Source: CAD feature listing. Evaluate the final solid. Frame: model axes, mm. A direction names the side the tool comes from. Coordinates: 2 decimals unless noted, no trailing zeros. Order: outer loops, then holes, each group sorted by start corner. A loop starts at its lowest first (then second) coordinate and runs counter-clockwise, first axis right, second up.
Item 1: Contact query for flat-ended pins moving along their axis: P1, Ø5.5, axis at x = 21, y = -2, coming from the +Z side; P2, Ø5, axis at x = -20.5, z = -1.5, coming from the -Y side; P3, Ø5, axis at y = -6.5, z = 3, coming from the +X side; P4, Ø5, axis at x = 11.5, y = -8, coming from the -Z side. Output: stop coordinate, or through.
Item 2: Section C-C on y = -8. Return the cut outline in (x, z).
Item 3: Section B-B on y = -2.5. Return the cut outline in (x, z).
Item 4: Section A-A on x = -28.5. Return the cut outline in (y, z), then the cut area to 3 significant figures.
Item 5: Reachability of faces 5 (the flat face through (24, -2, 3)), 6 (the flat face through (-15, -2, 3)), 7 (the flat face through (0, -2, -3)) from +Z, -Z, +X, -X, +Y, -Y: full face, straight path, thin tool, end or side. Return the list, or none.
Item 6: Section D-D on x = 22.5. Return the cut outline in (y, z).
Item 7: Ray query, line 1 (Z direction, x = 28.5, y = -3.55); line 2 (X direction, y = -3.25, z = 1); line 3 (X direction, y = -4.75, z = 1.75). Return the intervals inside material, ascending.
Item 8: Mould query, pull axis Z, two halves, no side actions, for faces 1 (the flat face through (6.207, -7.465, 1.257)), 2 (the cylindrical face through (8.359, -5.923, 3.31)), 3 (the cylindrical face through (30.646, -2.465, 0.676)), 4 (the flat face through (35.5, -2, 0)). Classes: released by +Z, released by -Z, zero draft, split by the parting line, or undercut.
from build123d import *

# Parameters (mm, degrees)
F0_R     = 2.25
F1_DEPTH = 5
F3_DEPTH = 5
F4_R     = 1.575
F5_DEPTH = 35.7601449816


with BuildPart() as f1:
    # F0 (on Front) → F1 (new body)
    with BuildSketch(Plane.XZ):
        Polygon((35.5, -3), (35.5, 3), (11.5355339059, 3), (8, -0.5355339059), (4.4644660941, 3), (-35.5, 3), (-35.5, -3), align=None)
        with Locations((-28.5, 0)):
            Circle(F0_R, mode=Mode.SUBTRACT)
        with Locations((28.5, 0)):
            Circle(F0_R, mode=Mode.SUBTRACT)
        Polygon((8, -0.5355339059), (11.5355339059, 3), (4.4644660941, 3), align=None)
        Polygon((4.4644660941, 3), (11.5355339059, 3), (8, 6.5355339059), align=None)
    extrude(amount=F1_DEPTH)

    # F2 (on face) → F3 (join)
    with BuildSketch(Plane.XZ.offset(5)):
        Polygon((11.5355339059, 3), (8, 6.5355339059), (4.4644660941, 3), (8, -0.5355339059), align=None)
    extrude(amount=F3_DEPTH)

    # F4 (on face) → F5 (cut, through all)
    with BuildSketch(Plane(origin=(4.267766953, 0, -4.267766953), x_dir=(0, 1, 0), z_dir=(0.7071067812, 0, -0.7071067812))):
        with Locations((-7.425, 7.7781745931)):
            Circle(F4_R)
    extrude(amount=-F5_DEPTH, mode=Mode.SUBTRACT)


solid = f1.part
Answer list:
1. P1: stops at z = 3
1. P2: stops at y = -5
1. P3: stops at x = 35.5
1. P4: stops at z = 0.56
2. outline: (4.46, 3) - (8, -0.54) - (8.73, 0.2) - (5.2, 3.73) - close; (7.27, 5.8) - (10.8, 2.27) - (11.54, 3) - (8, 6.54) - close
3. outline: (-35.5, -3) - (35.5, -3) - (35.5, 3) - (11.54, 3) - (8, 6.54) - (4.46, 3) - (-35.5, 3) - close; hole circle Ø4.5 at (-28.5, 0); hole circle Ø4.5 at (28.5, 0)
4. outline: (-5, -3) - (0, -3) - (0, -2.25) - (-5, -2.25) - close; (-5, 2.25) - (0, 2.25) - (0, 3) - (-5, 3) - close
4. area: 7.50 mm2
5. face 5: +Z, +X, +Y, -Y
5. face 6: +Z, -X, +Y, -Y
5. face 7: -Z, +X, -X, +Y, -Y
6. outline: (-5, -3) - (0, -3) - (0, 3) - (-5, 3) - close
7. line 1: z = -3 to -2.25, 2.25 to 3
7. line 2: x = -35.5 to -30.52, -26.48 to 26.48, 30.52 to 35.5
7. line 3: x = -35.5 to -29.91, -27.09 to 27.09, 29.91 to 35.5
8. face 1: released by -Z
8. face 2: undercut
8. face 3: undercut
8. face 4: zero draft
